from build123d import *

# Parameters (mm, degrees)
EXTRUDE_2_DEPTH      = 7
SKETCH_1_4_R         = 5
EXTRUDE_3_DEPTH      = 1.2
EXTRUDE_START        = 14
SKETCH_1_5_R         = 5
EXTRUDE_4_DEPTH      = 14
SKETCH_1_6_R         = 4.3
EXTRUDE_5_DEPTH      = 9
SKETCH_1_8_R         = 3.8
EXTRUDE_6_DEPTH      = 2
FILLET_1_R           = 1
CUT_EXTRUDE_START    = -2
SKETCH_1_10_R        = 1.6
CUT_EXTRUDE_31_DEPTH = 18.947831619
SKETCH_1_11_R        = 3
CUT_EXTRUDE_32_DEPTH = 7
CHAMFER_1_SIZE       = 0.5


with BuildPart() as part:
    # Эскиз1 → Бобышка-Вытянуть2 (new body)
    with BuildSketch(Plane.XY):
        Polygon((0, 5.773502692), (-5, 2.886751346), (-5, -2.886751346), (0, -5.773502692), (5, -2.886751346), (5, 2.886751346), align=None)
    extrude(amount=EXTRUDE_2_DEPTH)

    # Эскиз1<4> → Бобышка-Вытянуть3 (add)
    with BuildSketch(Plane.XY):
        Circle(SKETCH_1_4_R)
    extrude(amount=-EXTRUDE_3_DEPTH)

    # Эскиз1<5> → Бобышка-Вытянуть4 (add)
    with BuildSketch(Plane.XY.offset(EXTRUDE_START)):
        Circle(SKETCH_1_5_R)
    extrude(amount=-EXTRUDE_4_DEPTH)

    # Эскиз1<6> → Бобышка-Вытянуть5 (add)
    with BuildSketch(Plane.XY):
        Circle(SKETCH_1_6_R)
    extrude(amount=EXTRUDE_5_DEPTH)

    # Эскиз1<8> → Бобышка-Вытянуть6 (add)
    with BuildSketch(Plane.XY):
        Circle(SKETCH_1_8_R)
    extrude(amount=-EXTRUDE_6_DEPTH)

    # Скругление1
    fillet_1_edges = [part.edges().sort_by_distance(p)[0] for p in [
        (-5, 0, -1.2),
    ]]
    fillet(fillet_1_edges, radius=FILLET_1_R)

    # Эскиз1<10> → Вырез-Вытянуть31 (cut, through all)
    with BuildSketch(Plane.XY.offset(CUT_EXTRUDE_START)):
        Circle(SKETCH_1_10_R)
    extrude(amount=CUT_EXTRUDE_31_DEPTH, mode=Mode.SUBTRACT)

    # Эскиз1<11> → Вырез-Вытянуть32 (cut)
    with BuildSketch(Plane.XY.offset(CUT_EXTRUDE_START)):
        Circle(SKETCH_1_11_R)
    extrude(amount=CUT_EXTRUDE_32_DEPTH, mode=Mode.SUBTRACT)

    # Фаска1
    chamfer_1_edges = [part.edges().sort_by_distance(p)[0] for p in [
        (-5, 0, 14),
    ]]
    chamfer(chamfer_1_edges, length=CHAMFER_1_SIZE)


solid = part.part
Verification items for the finished model (mm, model axes). A direction names the side the tool comes from. Coordinates: 2 decimals unless noted, no trailing zeros. Order: outer loops, then holes, each group sorted by start corner. A loop starts at its lowest first (then second) coordinate and runs counter-clockwise, first axis right, second up. Notation, with made-up numbers: (87.25, 77.5) -> (97.25, 77.5) arc R21 ccw to (97.25, 102.5) -> close; hole circle Ø1 at (-16, -38). An arc over 180 degrees is marked (long way). Use CSV: the item, a comma, the result in double quotes. Start each with the question number.
Q1. Section check B-B, the plane z = 12.5. Record the cut outline in (x, y).
Q2. Draft check along X on faces 6 (the flat face through (-2.465, 4.35, 3.451)), 7 (the cylindrical face through (-1.27, -0.97, 9.44)), 8 (the flat face through (2.535, 4.31, 3.451)). Enter one of: +X half, -X half, draft (parallel to the pull), parting line (faces both ways), or undercut.
Q3. Tool access check on faces 1 (the cylindrical face through (-1.08, -4.88, 10.3)), 2 (the cylindrical face through (-3.796, 0.167, -1.594)), 3 (the flat face through (4.5, 2.7, 0)), 4 (the flat face through (0, -5.2, 7)), 5 (the flat face through (4.5, -2.6, 7)). Record the directions out of +Z, -Z, +X, -X, +Y, -Y that give a thin tool (end or side, any length) a straight path to the whole face; none if there is none.
Q4. Section check A-A, the plane z = 3.25. Record the cut outline in (x, y), and give its area (3 significant figures).
Q5. Thickness scan on line 1 along X through (y, z) = (0, 8); line 2 along Z through (x, y) = (-3.5, 1.75); line 3 along Z through (x, y) = (-1.25, 2.5). Record the ranges inside material, lowest first.
Q6. Depth check by flat-ended pin: P1, Ø2.5, axis at x = -3.5, y = -3, coming from the +Z side; P2, Ø1.2, axis at x = 4, y = -3, coming from the -Z side; P3, Ø2.5, axis at x = 1.5, y = 0, coming from the -Z side; P4, Ø2, axis at x = -2.5, z = 4, coming from the +Y side. Enter the tip coordinate at first touch or a pass-through.
Returned:
1,outline,"circle Ø10 at (0, 0); hole circle Ø3.2 at (0, 0)"
2,face 6,"-X half"
2,face 7,"undercut"
2,face 8,"+X half"
3,face 1,"+Z"
3,face 2,"-Z"
3,face 3,"-Z, +X, +Y"
3,face 4,"+Z, -Y"
3,face 5,"+Z, +X, -Y"
4,outline,"(-5, -2.89) -> (0, -5.77) -> (5, -2.89) -> (5, 2.89) -> (0, 5.77) -> (-5, 2.89) -> close; hole circle Ø6 at (0, 0)"
4,area,"58.3 mm^2"
5,line 1,"x = -5 to -1.6, 1.6 to 5"
5,line 2,"z = -1.2 to 14"
5,line 3,"z = 5 to 14"
6,P1,"stops at z = 14"
6,P2,"stops at z = -1.12"
6,P3,"stops at z = 5"
6,P4,"stops at y = 4.91"
